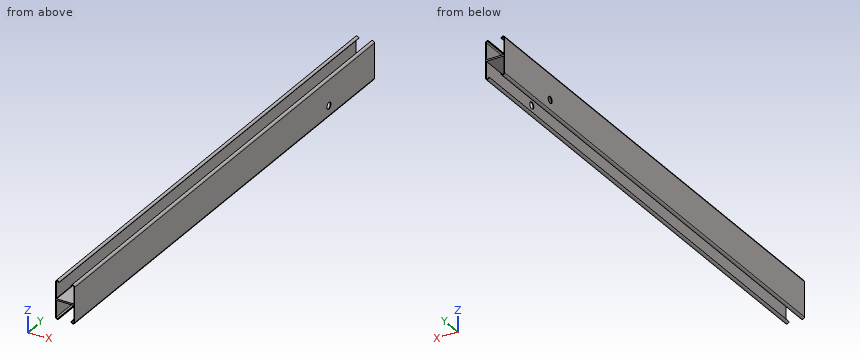
from build123d import *

# Parameters (mm, degrees)
F1_DEPTH = 533.4
F2_R     = 0.79374
F3_R     = 7.14375
F4_DEPTH = 41.276


# Not quite as in the source:
# - a fillet or chamfer is up to 0.001 mm smaller than in the source, because OpenCascade refuses the exact size


with BuildPart() as f1:
    # F0 (on Front) → F1 (new body, symmetric)
    with BuildSketch(Plane.XZ):
        with BuildLine():
            Line((0, 37.30625), (0, 0))
            Line((0, 0), (20.6375, 0))
            Line((20.6375, 0), (20.6375, 1.5875))
            Line((20.6375, 1.5875), (1.5875, 1.5875))
            Line((1.5875, 1.5875), (1.5875, 37.30625))
            ThreePointArc((1.5875, 37.30625), (3.96875, 39.6875), (6.35, 37.30625))
            Line((6.35, 37.30625), (7.9375, 37.30625))
            ThreePointArc((7.9375, 37.30625), (3.96875, 41.275), (0, 37.30625))
        make_face()
        with BuildLine():
            Line((20.6375, 0), (0, 0))
            Line((0, 0), (0, -37.30625))
            ThreePointArc((0, -37.30625), (3.96875, -41.275), (7.9375, -37.30625))
            Line((7.9375, -37.30625), (6.35, -37.30625))
            ThreePointArc((6.35, -37.30625), (3.96875, -39.6875), (1.5875, -37.30625))
            Line((1.5875, -37.30625), (1.5875, -1.5875))
            Line((1.5875, -1.5875), (20.6375, -1.5875))
            Line((20.6375, -1.5875), (20.6375, 0))
        make_face()
        with BuildLine():
            Line((20.6375, 1.5875), (20.6375, 0))
            Line((20.6375, 0), (41.275, 0))
            Line((41.275, 0), (41.275, 37.30625))
            ThreePointArc((41.275, 37.30625), (37.30625, 41.275), (33.3375, 37.30625))
            Line((33.3375, 37.30625), (34.925, 37.30625))
            ThreePointArc((34.925, 37.30625), (37.30625, 39.6875), (39.6875, 37.30625))
            Line((39.6875, 37.30625), (39.6875, 1.5875))
            Line((39.6875, 1.5875), (20.6375, 1.5875))
        make_face()
        with BuildLine():
            Line((41.275, 0), (20.6375, 0))
            Line((20.6375, 0), (20.6375, -1.5875))
            Line((20.6375, -1.5875), (39.6875, -1.5875))
            Line((39.6875, -1.5875), (39.6875, -37.30625))
            ThreePointArc((39.6875, -37.30625), (37.30625, -39.6875), (34.925, -37.30625))
            Line((34.925, -37.30625), (33.3375, -37.30625))
            ThreePointArc((33.3375, -37.30625), (37.30625, -41.275), (41.275, -37.30625))
            Line((41.275, -37.30625), (41.275, 0))
        make_face()
    extrude(amount=F1_DEPTH, both=True)

    # F2 (radius 0.79375 in the source; OpenCascade refuses exactly that, so slightly less here)
    f2_edges = [f1.edges().sort_by_distance(p)[0] for p in [
        (6.35, 0, 37.30625),
        (7.9375, 0, 37.30625),
        (33.3375, 0, 37.30625),
        (34.925, 0, 37.30625),
        (0, 0, 37.30625),
        (41.275, 0, 37.30625),
        (39.6875, 0, 1.5875),
        (1.5875, 0, 1.5875),
    ]]
    fillet(f2_edges, radius=F2_R)

    # F3 (on face) → F4 (cut, through all)
    with BuildSketch(Plane.YZ.offset(41.275)):
        with Locations((371.475, -16.66875)):
            Circle(F3_R)
    extrude(amount=-F4_DEPTH, mode=Mode.SUBTRACT)


solid = f1.part
Can you work these out from the model? Positions are in its coordinate system, mm. Round coordinates to 2 decimals unless told otherwise and drop trailing zeros. Write each loop counter-clockwise with the first axis right and the second up, starting at its lowest first coordinate (ties: lowest second). Pieces come first, ordered by that corner, then holes. Notation, with made-up numbers: (-6, -5) - (8, -5) arc R19 ccw to (8, 19) - close; hole circle Ø11 at (44, -25.5). An arc over 180 degrees is marked (long way). Write each question's results on one line, items separated by ' | '. Start each with the question number.
1) Suppose I cut it at A-A (z = 14). List the corners of the cut face in (x, y) for me (1 decimal).
2) Please list where these lines run through material, in increasing order: line 1 (Z direction, x = 7, y = -440.5); line 2 (X direction, y = 136.5, z = 12) (1 decimal); line 3 (X direction, y = -454.5, z = 38.5).
3) For pin 1 Ø0.5 at (x, y) = (7, 244.5) entering from +Z; pin 2 Ø18.5 at (x, y) = (16.5, -60) entering from +Z; pin 3 Ø11.5 at (x, y) = (12, 30) entering from -Z, each with a flat end and sliding along its axis, tell me the tip position at first contact or that it passes through.
4) Suppose I cut it at C-C (x = 22). List the corners of the cut face in (y, z) for me.
Here are the results:
1) outline: (0, -533.4) - (1.6, -533.4) - (1.6, 533.4) - (0, 533.4) - close; (39.7, -533.4) - (41.3, -533.4) - (41.3, 533.4) - (39.7, 533.4) - close
2) line 1: z = -39.87 to -37.31, -1.59 to 1.59, 37.31 to 39.87 | line 2: x = 0 to 1.6, 39.7 to 41.3 | line 3: x = 0.18 to 1.91, 6.03 to 7.75, 33.52 to 35.25, 39.37 to 41.09
3) pin 1: stops at z = 40.14 | pin 2: stops at z = 39.54 | pin 3: stops at z = -40.55
4) outline: (-533.4, -1.59) - (533.4, -1.59) - (533.4, 1.59) - (-533.4, 1.59) - close
